```python
from build123d import *

# Parameters (mm, degrees)
SKETCH1_R           = 4.5
BOSS_EXTRUDE1_DEPTH = 6.5
CUT_EXTRUDE1_DEPTH  = 6
CUT_EXTRUDE2_DEPTH  = 6


with BuildPart() as part:
    # Sketch1 → Boss-Extrude1 (new body, symmetric)
    with BuildSketch(Plane(origin=(0, 0, 0), x_dir=(1, 0, 0), z_dir=(0, 1, 0))):
        Circle(SKETCH1_R)
    extrude(amount=BOSS_EXTRUDE1_DEPTH, both=True)

    # Sketch2 → Cut-Extrude1 (cut)
    with BuildSketch(Plane.XZ.offset(6.5)):
        with BuildLine():
            Line((-1.5865, -2.115124996), (-1.5865, 2.115124996))
            ThreePointArc((-1.5865, 2.115124996), (0, 2.644), (1.5865, 2.115124996))
            Line((1.5865, 2.115124996), (1.5865, -2.115124996))
            ThreePointArc((1.5865, -2.115124996), (0, -2.644), (-1.5865, -2.115124996))
        make_face()
    extrude(amount=-CUT_EXTRUDE1_DEPTH, mode=Mode.SUBTRACT)

    # Sketch3 → Cut-Extrude2 (cut)
    with BuildSketch(Plane(origin=(0, 6.5, 0), x_dir=(1, 0, 0), z_dir=(0, 1, 0))):
        with BuildLine():
            Line((0.983, 2.433995892), (0.983, 1.683))
            ThreePointArc((0.983, 1.683), (1.188025253, 1.188025253), (1.683, 0.983))
            Line((1.683, 0.983), (2.433995892, 0.983))
            ThreePointArc((2.433995892, 0.983), (2.625, 0), (2.433995892, -0.983))
            Line((2.433995892, -0.983), (1.683, -0.983))
            ThreePointArc((1.683, -0.983), (1.188025253, -1.188025253), (0.983, -1.683))
            Line((0.983, -1.683), (0.983, -2.433995892))
            ThreePointArc((0.983, -2.433995892), (0, -2.625), (-0.983, -2.433995892))
            Line((-0.983, -2.433995892), (-0.983, -1.683))
            ThreePointArc((-0.983, -1.683), (-1.188025253, -1.188025253), (-1.683, -0.983))
            Line((-1.683, -0.983), (-2.433995892, -0.983))
            ThreePointArc((-2.433995892, -0.983), (-2.625, 0), (-2.433995892, 0.983))
            Line((-2.433995892, 0.983), (-1.683, 0.983))
            ThreePointArc((-1.683, 0.983), (-1.188025253, 1.188025253), (-0.983, 1.683))
            Line((-0.983, 1.683), (-0.983, 2.433995892))
            ThreePointArc((-0.983, 2.433995892), (0, 2.625), (0.983, 2.433995892))
        make_face()
    extrude(amount=-CUT_EXTRUDE2_DEPTH, mode=Mode.SUBTRACT)


solid = part.part
```
Input: part model. Units: mm. Frame: model coordinates. A direction names the side the tool comes from. Coordinates: 2 decimals unless noted, no trailing zeros. Write each loop counter-clockwise with the first axis right and the second up, starting at its lowest first coordinate (ties: lowest second). Pieces come first, ordered by that corner, then holes.
1) Section D-D on y = -2.5. Output: boundary loops of the cut face in (x, z).
2) Pin query (flat end, axial travel): pin 1 Ø0.8 at (y, z) = (3, -2) entering from +X; pin 2 Ø1.6 at (x, z) = (0, 0.5) entering from -Y; pin 3 Ø4 at (x, y) = (-3, 1) entering from -Z. Return the tip coordinate at first contact, or that it passes through.
3) Material intervals for line 1 along Z through (x, y) = (0, -2); line 2 along Z through (x, y) = (1.25, 3.75); line 3 along Y through (x, z) = (-0.25, -0.5), sorted ascending.
4) Section A-A on y = 3. Output: boundary loops of the cut face in (x, z) (3 decimals).
5) Section C-C on x = 0. Output: boundary loops of the cut face in (y, z) (3 decimals), and give its area (3 significant figures).
6) Mould query, pull axis X, two halves, no side actions, for faces 4 (the cylindrical face through (-0.59, 0.09, -4.46)), 5 (the flat face through (2, -6.5, 0)), 6 (the flat face through (0, 0.5, 0)). Classes: pulls with the +X half, pulls with the -X half, needs draft (parallel to the pull), parting line crosses it, or undercut.
7) Section B-B on z = 0. Output: boundary loops of the cut face in (x, y) (1 decimal), and give its area (3 significant figures).
8) Set-up query: faces 1 (the flat face through (0, -0.5, 0)), 2 (the flat face through (2, 6.5, 2)), 3 (the cylindrical face through (2.625, 3.542, -0.014)). Return all of +Z, -Z, +X, -X, +Y, -Y with unobstructed straight access to the full face (end or side cutting, diameter ignored); none if empty.
Check result:
1. outline: circle Ø9 at (0, 0); hole (-1.59, -2.12) arc R2.64 ccw to (1.59, -2.12) - (1.59, 2.12) arc R2.64 ccw to (-1.59, 2.12) - close
2. pin 1: stops at x = 4.21
2. pin 2: stops at y = -0.5
2. pin 3: stops at z = -4.39
3. line 1: z = -4.5 to -2.64, 2.64 to 4.5
3. line 2: z = -4.32 to -1.13, 1.13 to 4.32
3. line 3: y = -0.5 to 0.5
4. outline: circle Ø9 at (0, 0); hole (-2.434, -0.983) - (-1.683, -0.983) arc R0.7 cw to (-0.983, -1.683) - (-0.983, -2.434) arc R2.625 ccw to (0.983, -2.434) - (0.983, -1.683) arc R0.7 cw to (1.683, -0.983) - (2.434, -0.983) arc R2.625 ccw to (2.434, 0.983) - (1.683, 0.983) arc R0.7 cw to (0.983, 1.683) - (0.983, 2.434) arc R2.625 ccw to (-0.983, 2.434) - (-0.983, 1.683) arc R0.7 cw to (-1.683, 0.983) - (-2.434, 0.983) arc R2.625 ccw to start
5. outline: (-6.5, -4.5) - (6.5, -4.5) - (6.5, -2.625) - (0.5, -2.625) - (0.5, 2.625) - (6.5, 2.625) - (6.5, 4.5) - (-6.5, 4.5) - (-6.5, 2.644) - (-0.5, 2.644) - (-0.5, -2.644) - (-6.5, -2.644) - close
5. area: 53.8 mm2
6. face 4: parting line crosses it
6. face 5: needs draft
6. face 6: undercut
7. outline: (-4.5, -6.5) - (-1.6, -6.5) - (-1.6, -0.5) - (1.6, -0.5) - (1.6, -6.5) - (4.5, -6.5) - (4.5, 6.5) - (2.6, 6.5) - (2.6, 0.5) - (-2.6, 0.5) - (-2.6, 6.5) - (-4.5, 6.5) - close
7. area: 66.5 mm2
8. face 1: -Y
8. face 2: +Z, -Z, +X, -X, +Y
8. face 3: +Y
